CAD build for the part. Positions are in the model's coordinates, mm. A direction names the side the tool comes from. Give positions to 0.01 mm unless a question says otherwise; leave off trailing zeros. Write each loop counter-clockwise with the first axis right and the second up, starting at its lowest first coordinate (ties: lowest second). Pieces come first, ordered by that corner, then holes. Notation, with made-up numbers: (11, -9.5) - (21, -9.5) arc R30 cw to (21, 25.5) - close; hole circle Ø2 at (76.5, -38.5). An arc over 180 degrees is marked (long way). Write item = value, one per line. Start each with the question number.
```python
from build123d import *

# Parameters (mm, degrees)
ESBO_O1_R                = 1.6
ESBO_O1_W                = 65.5
ESBO_O1_H                = 5
RESSALTO_EXTRUS_O1_DEPTH = 4
ESBO_O2_W                = 5
ESBO_O2_H                = 10
RESSALTO_EXTRUS_O2_DEPTH = 10


with BuildPart() as part:
    # Esboço1 → Ressalto-extrusão1 (new body)
    with BuildSketch(Plane.XY):
        Polygon((-32.75, -2.5), (-32.75, -5), (-71.75, -5), (-71.75, 5), (-32.75, 5), (-32.75, 2.5), align=None)
        with Locations((-52.25, 0)):
            Circle(ESBO_O1_R, mode=Mode.SUBTRACT)
        with Locations((-67.75, 0)):
            Circle(ESBO_O1_R, mode=Mode.SUBTRACT)
        with Locations((-36.75, 0)):
            Circle(ESBO_O1_R, mode=Mode.SUBTRACT)
        Rectangle(ESBO_O1_W, ESBO_O1_H)
    extrude(amount=RESSALTO_EXTRUS_O1_DEPTH)

    # Esboço2 → Ressalto-extrusão2 (add)
    with BuildSketch(Plane.XY.offset(4)):
        with Locations((35.25, 0)):
            Rectangle(ESBO_O2_W, ESBO_O2_H)
    extrude(amount=-RESSALTO_EXTRUS_O2_DEPTH)


solid = part.part
```
1. Cut at C-C (z = -4.75). Give the cut face in (x, y).
2. Cut at D-D (x = 12.5). Give the cut face in (y, z).
3. Tool access for faces 4 (the flat face through (-32.75, -4, 2)), 5 (the flat face through (-32.75, 4, 2)), 6 (the flat face through (32.75, 0, -2)): list every direction of +Z, -Z, +X, -X, +Y, -Y with a clear straight run to the whole face (end or side of a thin tool).
4. Wall check: line 1 along X through (y, z) = (0.25, 2.25); line 2 along Y through (x, z) = (-52.25, 1.75); line 3 along Y through (x, z) = (30, 0.75). Give the ranges that are in metal, low to high.
5. Cut at A-A (y = 0). Give the cut face in (x, z).
6. Cut at B-B (x = -36.75). Give the cut face in (y, z), then the cut area to 3 significant figures.
7. Mould opens along X. For faces 1 (the flat face through (-71.75, 0, 2)), 2 (the flat face through (-30, 0, 0)), 3 (the cylindrical face through (-38, 1, 2)) say: +X half, -X half, draft (parallel to the pull), parting line (faces both ways), or undercut.
8. Pin check, flat tips, straight feed: pin 1 Ø6 at (x, y) = (-31.5, 1) entering from -Z; pin 2 Ø1.2 at (x, z) = (2, 2.5) entering from -Y; pin 3 Ø3 at (x, z) = (-50.5, -2) entering from -Y; pin 4 Ø1.2 at (x, z) = (4, 2) entering from +Y. Stop position of each tip, or through.
Output:
q1.outline = (32.75, -5) - (37.75, -5) - (37.75, 5) - (32.75, 5) - close
q2.outline = (-2.5, 0) - (2.5, 0) - (2.5, 4) - (-2.5, 4) - close
q3.face_4 = +Z, -Z, -Y
q3.face_5 = +Z, -Z, +Y
q3.face_6 = -Z
q4.line_1 = -71.75 to -69.33, -66.17 to -53.83, -50.67 to -38.33, -35.17 to 37.75
q4.line_2 = -5 to -1.6, 1.6 to 5
q4.line_3 = -2.5 to 2.5
q5.outline = (-71.75, 0) - (-69.35, 0) - (-69.35, 4) - (-71.75, 4) - close; (-66.15, 0) - (-53.85, 0) - (-53.85, 4) - (-66.15, 4) - close; (-50.65, 0) - (-38.35, 0) - (-38.35, 4) - (-50.65, 4) - close; (-35.15, 0) - (32.75, 0) - (32.75, -6) - (37.75, -6) - (37.75, 4) - (-35.15, 4) - close
q6.outline = (-5, 0) - (-1.6, 0) - (-1.6, 4) - (-5, 4) - close; (1.6, 0) - (5, 0) - (5, 4) - (1.6, 4) - close
q6.area = 27.2 mm2
q7.face_1 = -X half
q7.face_2 = draft
q7.face_3 = undercut
q8.pin_1 = 0
q8.pin_2 = -2.5
q8.pin_3 = through
q8.pin_4 = 2.5
